from build123d import *

# Parameters (mm, degrees)
SKETCH_1_W           = 86
SKETCH_1_H           = 86
EXTRUDE_1_DEPTH      = 2
SKETCH_2_R           = 3
CUT_EXTRUDE_1_DEPTH  = 3
SKETCH_3_R           = 3
CUT_EXTRUDE_2_DEPTH  = 3
SKETCH_4_R           = 3
CUT_EXTRUDE_3_DEPTH  = 3
SKETCH_6_R           = 3
CUT_EXTRUDE_4_DEPTH  = 3
SKETCH_7_R           = 3
CUT_EXTRUDE_5_DEPTH  = 3
SKETCH_8_R           = 3
CUT_EXTRUDE_6_DEPTH  = 3
SKETCH_9_R           = 3
CUT_EXTRUDE_7_DEPTH  = 3
SKETCH_10_R          = 3
CUT_EXTRUDE_8_DEPTH  = 3
SKETCH_11_R          = 3.290793372
CUT_EXTRUDE_9_DEPTH  = 3
SKETCH_12_W          = 6
SKETCH_12_H          = 6
CUT_EXTRUDE_10_DEPTH = 3
SKETCH_13_W          = 1
SKETCH_13_H          = 86
CUT_EXTRUDE_11_DEPTH = 3


with BuildPart() as part:
    # 草圖1 → 填料-伸長1 (new body)
    with BuildSketch(Plane.XY):
        with Locations((43, -43)):
            Rectangle(SKETCH_1_W, SKETCH_1_H)
    extrude(amount=EXTRUDE_1_DEPTH)

    # 草圖2 → 除料-伸長1 (cut)
    with BuildSketch(Plane.XY.offset(2)):
        with Locations((13, -13)):
            Circle(SKETCH_2_R)
    extrude(amount=-CUT_EXTRUDE_1_DEPTH, mode=Mode.SUBTRACT)

    # 草圖3 → 除料-伸長2 (cut)
    with BuildSketch(Plane.XY.offset(2)):
        with Locations((13, -45)):
            Circle(SKETCH_3_R)
    extrude(amount=-CUT_EXTRUDE_2_DEPTH, mode=Mode.SUBTRACT)

    # 草圖4 → 除料-伸長3 (cut)
    with BuildSketch(Plane.XY.offset(2)):
        with Locations((13, -76)):
            Circle(SKETCH_4_R)
    extrude(amount=-CUT_EXTRUDE_3_DEPTH, mode=Mode.SUBTRACT)

    # 草圖6 → 除料-伸長4 (cut)
    with BuildSketch(Plane.XY.offset(2)):
        with Locations((44, -8)):
            Circle(SKETCH_6_R)
    extrude(amount=-CUT_EXTRUDE_4_DEPTH, mode=Mode.SUBTRACT)

    # 草圖7 → 除料-伸長5 (cut)
    with BuildSketch(Plane.XY.offset(2)):
        with Locations((44, -78)):
            Circle(SKETCH_7_R)
    extrude(amount=-CUT_EXTRUDE_5_DEPTH, mode=Mode.SUBTRACT)

    # 草圖8 → 除料-伸長6 (cut)
    with BuildSketch(Plane.XY.offset(2)):
        with Locations((60, -34)):
            Circle(SKETCH_8_R)
    extrude(amount=-CUT_EXTRUDE_6_DEPTH, mode=Mode.SUBTRACT)

    # 草圖9 → 除料-伸長7 (cut)
    with BuildSketch(Plane.XY.offset(2)):
        with Locations((60, -47)):
            Circle(SKETCH_9_R)
    extrude(amount=-CUT_EXTRUDE_7_DEPTH, mode=Mode.SUBTRACT)

    # 草圖10 → 除料-伸長8 (cut)
    with BuildSketch(Plane.XY.offset(2)):
        with Locations((60, -59)):
            Circle(SKETCH_10_R)
    extrude(amount=-CUT_EXTRUDE_8_DEPTH, mode=Mode.SUBTRACT)

    # 草圖11 → 除料-伸長9 (cut)
    with BuildSketch(Plane.XY.offset(2)):
        with Locations((60, -74)):
            Circle(SKETCH_11_R)
    extrude(amount=-CUT_EXTRUDE_9_DEPTH, mode=Mode.SUBTRACT)

    # 草圖12 → 除料-伸長10 (cut)
    with BuildSketch(Plane.XY.offset(2)):
        with Locations((38, -31)):
            Rectangle(SKETCH_12_W, SKETCH_12_H)
    extrude(amount=-CUT_EXTRUDE_10_DEPTH, mode=Mode.SUBTRACT)

    # 草圖13 → 除料-伸長11 (cut)
    with BuildSketch(Plane.XY.offset(2)):
        with Locations((85.5, -43)):
            Rectangle(SKETCH_13_W, SKETCH_13_H)
        with Locations((0.5, -43)):
            Rectangle(SKETCH_13_W, SKETCH_13_H)
    extrude(amount=-CUT_EXTRUDE_11_DEPTH, mode=Mode.SUBTRACT)


solid = part.part
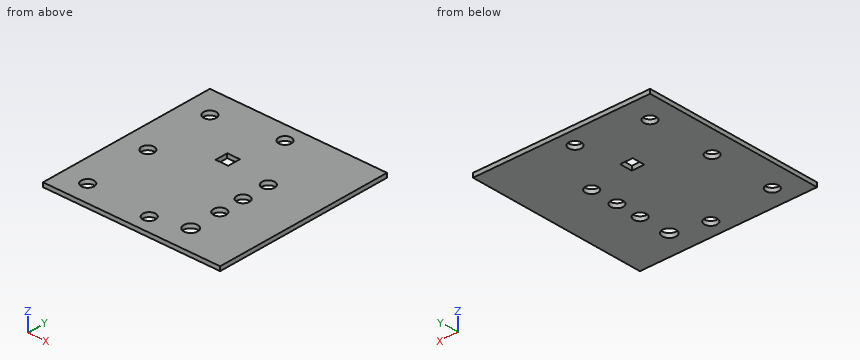
Design review of the part built by this model. Coordinates are the model's own, in mm. Round coordinates to 2 decimals unless told otherwise and drop trailing zeros. Write each loop counter-clockwise with the first axis right and the second up, starting at its lowest first coordinate (ties: lowest second). Pieces come first, ordered by that corner, then holes. Notation, with made-up numbers: M 2.25,33.5 L 25.25,33.5 A30 cw 25.25,63.5 Z; hole C 89,76.25 d5. An arc over 180 degrees is marked long. One line per item, written item: value. Start each with the question number.
1. Take a section at D-D on z = 0.5. State how many separate pieces and enclosed holes the cut face has, then the cut area to 3 significant figures.
2. Take a section at B-B on y = -59. State the section outline as (x, z) points, then the cut area to 3 significant figures.
3. Take a section at C-C on x = 44. State the section outline as (y, z) points, then the cut area to 3 significant figures.
4. To check wall thickness, follow probe 1 along Y at (x, z) = (44, 1.35); probe 2 along Y at (x, z) = (60, 1.4); probe 3 along Y at (x, z) = (13, 1). State the ranges of each line that lie inside material, in increasing order. Write a range as from..to.
5. Take a section at A-A on x = 13. State the section outline as (y, z) points.
Computed:
1. separate pieces: 1
1. enclosed holes: 10
1. area: 6,930 mm²
2. outline: M 1,0 L 57,0 L 57,2 L 1,2 Z; M 63,0 L 85,0 L 85,2 L 63,2 Z
2. area: 156 mm²
3. outline: M -86,0 L -81,0 L -81,2 L -86,2 Z; M -75,0 L -11,0 L -11,2 L -75,2 Z; M -5,0 L 0,0 L 0,2 L -5,2 Z
3. area: 148 mm²
4. probe 1: y = -86..-81, -75..-11, -5..0
4. probe 2: y = -86..-77.29, -70.71..-62, -56..-50, -44..-37, -31..0
4. probe 3: y = -86..-79, -73..-48, -42..-16, -10..0
5. outline: M -86,0 L -79,0 L -79,2 L -86,2 Z; M -73,0 L -48,0 L -48,2 L -73,2 Z; M -42,0 L -16,0 L -16,2 L -42,2 Z; M -10,0 L 0,0 L 0,2 L -10,2 Z
